Geometry: final body of the model. Coordinates: model frame, mm. Coordinates: 2 decimals unless noted, no trailing zeros. Write each loop counter-clockwise with the first axis right and the second up, starting at its lowest first coordinate (ties: lowest second). Pieces come first, ordered by that corner, then holes. Notation, with made-up numbers: M -27.5,-4.75 L 6.5,-4.75 A28 ccw 6.5,20.25 Z; hole C -21,75.25 d6. An arc over 180 degrees is marked long. Write item = value, one per line. Start each with the question number.
Item 1: Section A-A on z = 47. Output: boundary loops of the cut face in (x, y), plus the area to 3 significant figures.
Item 2: First-contact query: pin 1 Ø10 at (x, z) = (-34.5, 62) entering from -Y; pin 2 Ø12 at (x, z) = (45, 53.5) entering from -Y; pin 3 Ø5 at (x, z) = (-20, 36) entering from +Y. Flat tips, straight axial feed; report the tip coordinate or a pass-through.
Item 3: Pull-direction query (Y, two-part tool) for faces 1 (the flat face through (13, -59, -100)), 2 (the cylindrical face through (-62.44, 2.75, 1.39)), 3 (the cylindrical face through (-59.94, 2.64, -1.4)); classes: +Y half, -Y half, draft (parallel to the pull), parting line (faces both ways), or undercut.
Item 4: Ray query, L1, parallel to Y at x = 2.5, z = -64; L2, parallel to Z at x = 0, y = -61; L3, parallel to Y at x = 33, z = -11. Return the intervals inside material, ascending. Write a range as [from, to].
from build123d import *

# Parameters (mm, degrees)
SKETCH1_R           = 62.5
SKETCH1_R_2         = 60
BOSS_EXTRUDE1_DEPTH = 100
SKETCH2_R           = 2
CUT_EXTRUDE1_DEPTH  = 100
SKETCH3_R           = 2
CUT_EXTRUDE2_DEPTH  = 74
CHAMFER1_SIZE       = 1
CHAMFER2_SIZE       = 1


with BuildPart() as part:
    # Sketch1 → Boss-Extrude1 (new, symmetric)
    with BuildSketch(Plane.XY):
        Circle(SKETCH1_R)
        Circle(SKETCH1_R_2, mode=Mode.SUBTRACT)
    extrude(amount=BOSS_EXTRUDE1_DEPTH, both=True)

    # Sketch2 → Cut-Extrude1 (cut, symmetric)
    with BuildSketch(Plane(origin=(0, 0, 0), x_dir=(1, 0, 0), z_dir=(0, 1, 0))):
        with Locations(Location((0, -30, 0), (0, 0, 270))):
            Circle(SKETCH2_R)
    extrude(amount=CUT_EXTRUDE1_DEPTH, both=True, mode=Mode.SUBTRACT)

    # Sketch3 → Cut-Extrude2 (cut, symmetric)
    with BuildSketch(Plane(origin=(0, 0, 0), x_dir=(0, 0, -1), z_dir=(1, 0, 0))):
        with Locations((-30, 0)):
            Circle(SKETCH3_R)
    extrude(amount=CUT_EXTRUDE2_DEPTH, both=True, mode=Mode.SUBTRACT)

    # Chamfer1
    chamfer1_edges = [part.edges().sort_by_distance(p)[0] for p in [
        (-62.5, 0, 100),
    ]]
    chamfer(chamfer1_edges, length=CHAMFER1_SIZE)

    # Chamfer2
    chamfer2_edges = [part.edges().sort_by_distance(p)[0] for p in [
        (-62.5, 0, -100),
    ]]
    chamfer(chamfer2_edges, length=CHAMFER2_SIZE)


solid = part.part
Responses:
q1.outline = C 0,0 d125; hole C 0,0 d120
q1.area = 962 mm²
q2.pin_1 = -55.1
q2.pin_2 = -48.84
q2.pin_3 = 60
q3.face_1 = draft
q3.face_2 = parting line
q3.face_3 = undercut
q4.L1 = [-62.45, -59.95], [59.95, 62.45]
q4.L2 = [-100, 28], [32, 100]
q4.L3 = [-53.08, -50.11], [50.11, 53.08]
